The model under review builds one solid part; all positions refer to its coordinate system, in mm. A direction names the side the tool comes from. Round coordinates to 2 decimals unless told otherwise and drop trailing zeros. Order: outer loops, then holes, each group sorted by start corner. A loop starts at its lowest first (then second) coordinate and runs counter-clockwise, first axis right, second up. Notation, with made-up numbers: M 35,-24.75 L 50,-24.75 A17 ccw 50,-3.75 Z; hole C 6,61.25 d5. An arc over 180 degrees is marked long. Use a Markdown table: item, result. Add a question column.
1. The part is to be moulded in two halves that separate along Y. For faces 1 (the flat face through (28, 47.805, 19)), 2 (the flat face through (28, 20.805, 29)), 3 (the flat face through (17.077, 32, 19)), say which applies: +Y half, -Y half, draft (parallel to the pull), parting line (faces both ways), or undercut.
2. Consider section D-D on y = 36.5. State the section outline as (x, z) points, then the cut area to 3 significant figures.
3. Consider section B-B on x = 25.5. State the section outline as (y, z) points, then the cut area to 3 significant figures.
4. Insertion check: P1, Ø9.5, axis at x = 28, y = 31.5, coming from the -Z side; P2, Ø8, axis at x = 29.5, y = 26, coming from the +Z side; P3, Ø2, axis at y = 38, z = 101.5, coming from the -X side. Each pin has a flat end and moves straight along its axis. Give the tip position at first contact, or say it passes through.
5. Consider section C-C on y = 25.5. State the section outline as (x, z) points, then the cut area to 3 significant figures.
6. To check wall thickness, follow probe 1 along Y at (x, z) = (27.75, 35); probe 2 along X at (y, z) = (21.5, -19); probe 3 along Z at (x, y) = (25.5, 31). State the ranges of each line that lie inside material, in increasing order.
7. For faces 4 (the flat face through (21, 32, -60)), 5 (the flat face through (34.077, 32, 19)), 6 (the flat face through (28, 34.839, -43)), 7 (the flat face through (19.077, 25, 101)), list the 3-axis set-ups (+Z, -Z, +X, -X, +Y, -Y) from which the entire face can be reached by the end or side of a thin tool; tool diameter is ignored.
8. Consider section A-A on z = 21. State the section outline as (x, y) points.
Autodesk Inventor part; units mm, degrees
ref_plane "YZ Plane" through (0, 0, 0) normal (1, 0, 0) x (0, 1, 0)
ref_plane "XZ Plane" through (0, 0, 0) normal (0, 1, 0) x (-1, 0, 0)
ref_plane "XY Plane" through (0, 0, 0) normal (0, 0, 1) x (1, 0, 0)
sketch "Sketch1" plane through (0, 0, 0) normal (0, 0, 1) x (1, 0, 0)
  line L0 (22.0768, 42.8051) -> (34.0768, 42.8051)
  line L1 (34.0768, 42.8051) -> (34.0768, 20.8051)
  line L2 (34.0768, 20.8051) -> (22.0768, 20.8051)
  line L3 (22.0768, 20.8051) -> (22.0768, 42.8051)
  line L4 (39.0768, 47.8051) -> (17.0768, 47.8051)
  line L5 (17.0768, 47.8051) -> (17.0768, 15.8051)
  line L6 (17.0768, 15.8051) -> (39.0768, 15.8051)
  line L7 (39.0768, 15.8051) -> (39.0768, 47.8051)
  line L8 (34.0768, 20.8051) -> (34.0768, 15.8051)
  line L9 (22.0768, 20.8051) -> (22.0768, 15.8051)
  line L10 (22.0768, 42.8051) -> (22.0768, 47.8051)
  line L11 (34.0768, 42.8051) -> (34.0768, 47.8051)
  point P0 (0, 0)
  dimension "d4" = 12
  dimension "d5" = 22
  dimension "d6" = 5
extrude "Extrusion2" add sketch "Sketch1" along normal blind 100 and the other way blind 60 contours L10 L4 L11 L0 | L3 L9 L6 L5 L4 L10 | L11 L4 L7 L6 L8 L1 | L2 L8 L6 L9
sketch "Sketch2" plane through (39.0768, 15.8051, 100) normal (1, 0, 0) x (0, 0, -1)
  line L0 (0, 0) -> (0, 32)
  line L1 (0, 0) -> (30.1146, 0) construction
  line L2 (0, 32) -> (-2.7996, 0)
  line L3 (0, 32) -> (32.6362, 32) construction
  line L4 (0, 0) -> (-2.7996, 0)
  point P0 (100, -15.8051)
  dimension "d16" = 95
extrude "Extrusion3" add sketch "Sketch2" against normal blind 20
sketch "Sketch3" plane through (0, 0, -60) normal (0, 0, -1) x (-1, 0, 0)
  line L0 (-17.0768, 15.8051) -> (-37.0768, 15.8051)
  line L1 (-37.0768, 15.8051) -> (-37.0768, 36.9275)
  line L2 (-37.0768, 36.9275) -> (-17.0768, 36.9275)
  line L3 (-17.0768, 36.9275) -> (-17.0768, 15.8051)
  line L4 (-22.0768, 20.8051) -> (-34.0768, 20.8051)
  line L5 (-34.0768, 20.8051) -> (-34.0768, 34.8394)
  line L6 (-34.0768, 34.8394) -> (-22.0768, 34.8394)
  line L7 (-22.0768, 34.8394) -> (-22.0768, 20.8051)
  point P0 (0, 0)
  dimension "d17" = 20
  dimension "d18" = 12
extrude "Extrusion4" add sketch "Sketch3" against normal blind 20 contours L4 L5 L6 L7
extrude "Extrusion5" cut sketch "Sketch3" against normal blind 15 contours L4 L5 L6 L7
properties part number "motorstand2"
Answer block:
| question | item | result |
|---|---|---|
| 1 | face 1 | +Y half |
| 1 | face 2 | undercut |
| 1 | face 3 | draft |
| 2 | outline | M 17.08,-60 L 22.08,-60 L 22.08,100 L 34.08,100 L 34.08,-60 L 39.08,-60 L 39.08,100.99 L 19.08,100.99 L 19.08,100 L 17.08,100 Z |
| 2 | area | 1,620 mm^2 |
| 3 | outline | M 15.81,-60 L 20.81,-60 L 20.81,-45 L 34.84,-45 L 34.84,-40 L 20.81,-40 L 20.81,100 L 42.81,100 L 42.81,-60 L 47.81,-60 L 47.81,100 L 15.81,102.8 Z |
| 3 | area | 1,710 mm^2 |
| 4 | P1 | z = -45 |
| 4 | P2 | z = 102.26 |
| 4 | P3 | x = 19.08 |
| 5 | outline | M 17.08,-60 L 22.08,-60 L 22.08,-45 L 34.08,-45 L 34.08,-60 L 39.08,-60 L 39.08,101.95 L 19.08,101.95 L 19.08,100 L 17.08,100 Z; hole M 22.08,-40 L 34.08,-40 L 34.08,100 L 22.08,100 Z |
| 5 | area | 1,700 mm^2 |
| 6 | probe 1 | 15.81 to 20.81, 42.81 to 47.81 |
| 6 | probe 2 | 17.08 to 22.08, 34.08 to 39.08 |
| 6 | probe 3 | -45 to -40, 100 to 101.47 |
| 7 | face 4 | -Z, +X, -X, +Y, -Y |
| 7 | face 5 | none |
| 7 | face 6 | -Z |
| 7 | face 7 | +Z, -X, +Y, -Y |
| 8 | outline | M 17.08,15.81 L 39.08,15.81 L 39.08,47.81 L 17.08,47.81 Z; hole M 22.08,20.81 L 34.08,20.81 L 34.08,42.81 L 22.08,42.81 Z |
